```python
from build123d import *

# Parameters (mm, degrees)
SKETCH_1_W          = 218
SKETCH_1_H          = 218
EXTRUDE_1_DEPTH     = 4
FILLET_1_R          = 4
SKETCH_2_R          = 1.5
CUT_EXTRUDE_3_DEPTH = 2.2
SKETCH_2_3_R        = 1.5
CUT_EXTRUDE_4_DEPTH = 155.201167311


with BuildPart() as part:
    # Sketch 1 → Extrude 1 (new body)
    with BuildSketch(Plane(origin=(0, 0, 0), x_dir=(1, 0, 0), z_dir=(0, 1, 0))):
        Rectangle(SKETCH_1_W, SKETCH_1_H)
    extrude(amount=EXTRUDE_1_DEPTH)

    # Fillet 1
    fillet_1_edges = [part.edges().sort_by_distance(p)[0] for p in [
        (-109, 2, -109),
        (109, 2, -109),
        (109, 2, 109),
        (-109, 2, 109),
    ]]
    fillet(fillet_1_edges, radius=FILLET_1_R)

    # Sketch 2 → Cut-Extrude 3 (cut)
    # profile 1 of 4: a face of its own
    with BuildSketch(Plane(origin=(0, 4, 0), x_dir=(1, 0, 0), z_dir=(0, 1, 0))):
        Polygon((105.375169377, 106.862209377), (102.208838657, 106.622036303), (100.83366928, 103.759826926), (102.624830623, 101.137790623), (105.791161343, 101.377963697), (107.16633072, 104.240173074), align=None)
        with Locations(Location((104, 104, 0), (0, 0, 270))):
            Circle(SKETCH_2_R, mode=Mode.SUBTRACT)
    # profile 2 of 4: a face of its own
    with BuildSketch(Plane(origin=(0, 4, 0), x_dir=(1, 0, 0), z_dir=(0, 1, 0))):
        Polygon((107.16633072, -104.240173074), (105.375169377, -106.862209377), (102.208838657, -106.622036303), (100.83366928, -103.759826926), (102.624830623, -101.137790623), (105.791161343, -101.377963697), align=None)
        with Locations(Location((104, -104, 0), (0, 0, 270))):
            Circle(SKETCH_2_R, mode=Mode.SUBTRACT)
    # profile 3 of 4: a face of its own
    with BuildSketch(Plane(origin=(0, 4, 0), x_dir=(1, 0, 0), z_dir=(0, 1, 0))):
        Polygon((-107.16633072, -104.240173074), (-105.375169377, -106.862209377), (-102.208838657, -106.622036303), (-100.83366928, -103.759826926), (-102.624830623, -101.137790623), (-105.791161343, -101.377963697), align=None)
        with Locations(Location((-104, -104, 0), (0, 0, 270))):
            Circle(SKETCH_2_R, mode=Mode.SUBTRACT)
    # profile 4 of 4: a face of its own
    with BuildSketch(Plane(origin=(0, 4, 0), x_dir=(1, 0, 0), z_dir=(0, 1, 0))):
        Polygon((-105.791161343, 101.377963697), (-107.16633072, 104.240173074), (-105.375169377, 106.862209377), (-102.208838657, 106.622036303), (-100.83366928, 103.759826926), (-102.624830623, 101.137790623), align=None)
        with Locations(Location((-104, 104, 0), (0, 0, 270))):
            Circle(SKETCH_2_R, mode=Mode.SUBTRACT)
    extrude(amount=-CUT_EXTRUDE_3_DEPTH, mode=Mode.SUBTRACT)

    # Sketch 2_3 → Cut-Extrude 4 (cut, through all)
    with BuildSketch(Plane(origin=(0, 4, 0), x_dir=(1, 0, 0), z_dir=(0, 1, 0))):
        with Locations(Location((104, -104, 0), (0, 0, 270))):
            Circle(SKETCH_2_3_R)
        with Locations(Location((-104, -104, 0), (0, 0, 270))):
            Circle(SKETCH_2_3_R)
        with Locations(Location((-104, 104, 0), (0, 0, 270))):
            Circle(SKETCH_2_3_R)
        with Locations(Location((104, 104, 0), (0, 0, 270))):
            Circle(SKETCH_2_3_R)
    extrude(amount=-CUT_EXTRUDE_4_DEPTH, mode=Mode.SUBTRACT)


solid = part.part
```
Verification items for the finished model (mm, model axes). A direction names the side the tool comes from. Round coordinates to 2 decimals unless told otherwise and drop trailing zeros. Answer as a JSON object with one key per item and string values.
Q1. Access from +Z, -Z, +X, -X, +Y, -Y to the whole of each face (thin tool, end or side, straight path). Record for faces 3 (the flat face through (105.5, 1.8, 103.3)), 4 (the flat face through (-2, 4, -2)).
Data:
{"face 3": "+Y", "face 4": "+Z, -Z, +X, -X, +Y"}
Q2. Scan line: line 1 (X direction, y = 0.7, z = -104). Record every from-to range of solid material in increasing order. Write a range as from..to.
Data:
{"line 1": "x = -109..-105.5, -102.5..102.5, 105.5..109"}
Q3. Draft check along X on faces 1 (the flat face through (-2, 0, -2)), 2 (the flat face through (-102.5, 1.8, -104.7)). Enter one of: pulls with the +X half, pulls with the -X half, needs draft (parallel to the pull), parting line crosses it, or undercut.
Data:
{"face 1": "needs draft", "face 2": "undercut"}
Q4. Go/stop test with a flat-tipped pin: P1, Ø1.7, axis at x = 102.5, z = 104.5, coming from the +Y side. Record where the tip stops, or that it passes through.
Data:
{"P1": "stops at y = 1.8"}
